```python
from build123d import *

# Parameters (mm, degrees)
HIERRO_ANGULAR_2_X_2_X_0_125_1_DEPTH = 38.1


with BuildPart() as part:
    # Sketch12 → Hierro angular 2 X 2 X 0.125(1) (new body)
    with BuildSketch(Plane.YZ):
        with BuildLine():
            Line((0, 0), (0, 50.8))
            Line((0, 50.8), (0.00508, 50.8))
            ThreePointArc((0.00508, 50.8), (2.246551928, 49.871551928), (3.175, 47.63008))
            Line((3.175, 47.63008), (3.175, 7.9375))
            ThreePointArc((3.175, 7.9375), (4.569903955, 4.569903955), (7.9375, 3.175))
            Line((7.9375, 3.175), (47.63008, 3.175))
            ThreePointArc((47.63008, 3.175), (49.871551928, 2.246551928), (50.8, 0.00508))
            Line((50.8, 0.00508), (50.8, 0))
            Line((50.8, 0), (0, 0))
        make_face()
    extrude(amount=HIERRO_ANGULAR_2_X_2_X_0_125_1_DEPTH)


solid = part.part
```
The listing builds one solid part. Answer for the finished solid, in the listing's coordinates (mm). A direction names the side the tool comes from. Round coordinates to 2 decimals unless told otherwise and drop trailing zeros. Order: outer loops, then holes, each group sorted by start corner. A loop starts at its lowest first (then second) coordinate and runs counter-clockwise, first axis right, second up. Notation, with made-up numbers: (7.25, -24) -> (50.25, -24) arc R5 ccw to (50.25, -18) -> close; hole circle Ø1 at (-24, -21.75). An arc over 180 degrees is marked (long way). Answer as CSV lines item,"result". Start each with the question number.
(1) Flat-ended cylindrical pins translate along their axes: pin 1 Ø11.5 at (x, y) = (12, 24) entering from +Z (3 decimals); pin 2 Ø10 at (x, y) = (5, 45) entering from -Z; pin 3 Ø19 at (x, z) = (17.5, 29.5) entering from +Y (3 decimals). Find the tip coordinate at first contact, or state that the pin passes through.
(2) The part is cut by section B-B (y = 23). Determine the outline of the cut face in (x, z) (3 decimals), then the cut area to 3 significant figures.
(3) Find the intervals of material crossed by probe 1 along Z at (x, y) = (9, 16.5) (3 decimals); probe 2 along Z at (x, y) = (3.5, 4), in increasing order. Write a range as from..to.
(4) A tool of negligible diameter and unlimited length cuts with its end or side. For faces 1 (the face through (38.1, 14, 3)), 2 (the face through (19, 3.175, 28)), from which of +Z, -Z, +X, -X, +Y, -Y can it reach the whole face along a straight path? Write none if from no direction.
Evaluation:
1,pin 1,"z = 3.175"
1,pin 2,"z = 0"
1,pin 3,"y = 3.175"
2,outline,"(0, 0) -> (38.1, 0) -> (38.1, 3.175) -> (0, 3.175) -> close"
2,area,"121 mm²"
3,probe 1,"0..3.175"
3,probe 2,"0..5.26"
4,face 1,"+Z, -Z, +X, +Y, -Y"
4,face 2,"+Z, +X, -X, +Y"
